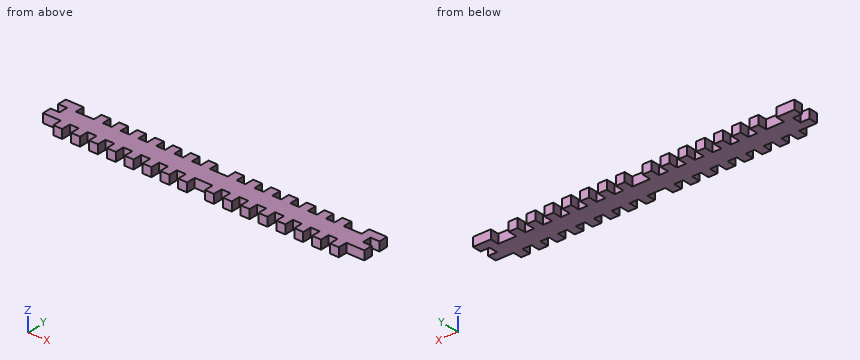
from build123d import *

# Parameters (mm, degrees)
BOSS_EXTRUDE1_DEPTH = 6.35


with BuildPart() as part:
    # Sketch1 → Boss-Extrude1 (new body)
    with BuildSketch(Plane.XY):
        Polygon((-107.95, 0), (-114.3, 0), (-114.3, -6.35), (-101.6, -6.35), (-101.6, -12.7), (-95.25, -12.7), (-95.25, -6.35), (-88.9, -6.35), (-88.9, -12.7), (-82.55, -12.7), (-82.55, -6.35), (-76.2, -6.35), (-76.2, -12.7), (-69.85, -12.7), (-69.85, -6.35), (-63.5, -6.35), (-63.5, -12.7), (-57.15, -12.7), (-57.15, -6.35), (-50.8, -6.35), (-50.8, -12.7), (-44.45, -12.7), (-44.45, -6.35), (-38.1, -6.35), (-38.1, -12.7), (-31.75, -12.7), (-31.75, -6.35), (-25.4, -6.35), (-25.4, -12.7), (-19.05, -12.7), (-19.05, -6.35), (-12.7, -6.35), (-12.7, -12.7), (-6.35, -12.7), (-6.35, -6.35), (0, -6.35), (6.35, -6.35), (6.35, -12.7), (12.7, -12.7), (12.7, -6.35), (19.05, -6.35), (19.05, -12.7), (25.4, -12.7), (25.4, -6.35), (31.75, -6.35), (31.75, -12.7), (38.1, -12.7), (38.1, -6.35), (44.45, -6.35), (44.45, -12.7), (50.8, -12.7), (50.8, -6.35), (57.15, -6.35), (57.15, -12.7), (63.5, -12.7), (63.5, -6.35), (69.85, -6.35), (69.85, -12.7), (76.2, -12.7), (76.2, -6.35), (82.55, -6.35), (82.55, -12.7), (88.9, -12.7), (88.9, -6.35), (95.25, -6.35), (95.25, -12.7), (101.6, -12.7), (101.6, -6.35), (114.3, -6.35), (114.3, 0), (107.95, 0), (107.95, 6.35), (114.3, 6.35), (114.3, 12.7), (107.95, 12.7), (101.6, 12.7), (101.6, 6.35), (95.25, 6.35), (88.9, 6.35), (88.9, 12.7), (82.55, 12.7), (82.55, 6.35), (76.2, 6.35), (76.2, 12.7), (69.85, 12.7), (69.85, 6.35), (63.5, 6.35), (63.5, 12.7), (57.15, 12.7), (57.15, 6.35), (50.8, 6.35), (50.8, 12.7), (44.45, 12.7), (44.45, 6.35), (38.1, 6.35), (38.1, 12.7), (31.75, 12.7), (31.75, 6.35), (25.4, 6.35), (25.4, 12.7), (19.05, 12.7), (19.05, 6.35), (12.7, 6.35), (12.7, 12.7), (6.35, 12.7), (6.35, 6.35), (0, 6.35), (-6.35, 6.35), (-6.35, 12.7), (-12.7, 12.7), (-12.7, 6.35), (-19.05, 6.35), (-19.05, 12.7), (-25.4, 12.7), (-25.4, 6.35), (-31.75, 6.35), (-31.75, 12.7), (-38.1, 12.7), (-38.1, 6.35), (-44.45, 6.35), (-44.45, 12.7), (-50.8, 12.7), (-50.8, 6.35), (-57.15, 6.35), (-57.15, 12.7), (-63.5, 12.7), (-63.5, 6.35), (-69.85, 6.35), (-69.85, 12.7), (-76.2, 12.7), (-76.2, 6.35), (-82.55, 6.35), (-82.55, 12.7), (-88.9, 12.7), (-88.9, 6.35), (-95.25, 6.35), (-101.6, 6.35), (-101.6, 12.7), (-107.95, 12.7), (-114.3, 12.7), (-114.3, 6.35), (-107.95, 6.35), align=None)
    extrude(amount=BOSS_EXTRUDE1_DEPTH)


solid = part.part
Design review of the part built by this model. Coordinates are the model's own, in mm. Coordinates: 2 decimals unless noted, no trailing zeros. Loops run counter-clockwise (first coordinate to the right, second up) from the corner with the lowest first, then second, coordinate; pieces in that order, holes last. Notation, with made-up numbers: (32.5, 72) - (42.5, 72) arc R14 ccw to (42.5, 93) - close; hole circle Ø9 at (82.25, -13.5). An arc over 180 degrees is marked (long way). Use CSV: the item, a comma, the result in double quotes. Start each with the question number.
1. To check wall thickness, follow probe 1 along X at (y, z) = (2, 2); probe 2 along Y at (x, z) = (-99.5, 2.5); probe 3 along Y at (x, z) = (-15, 4.75). State the ranges of each line that lie inside material, in increasing order.
2. Clearance check with flat-ended pins moving along their axes: pin 1 (1.9 mm diameter, centred on x = 91, z = 2, fed in from -Y); pin 2 (3 mm diameter, centred on y = -9, z = 3.5, fed in from -X); pin 3 (1 mm diameter, centred on y = 5.5, z = 3, fed in from +X). State where each tip first meets the part, or that it passes through.
3. Add section A-A on y = 8.75. Count the separate pieces of the cut face and the enclosed holes in it, plus the area to 3 significant figures.
4. Add section B-B on x = 53.5. Give the boundary of the cut face in (y, z).
Resolved:
1,probe 1,"-107.95 to 107.95"
1,probe 2,"-12.7 to 6.35"
1,probe 3,"-6.35 to 6.35"
2,pin 1,"y = -6.35"
2,pin 2,"x = -101.6"
2,pin 3,"x = 107.95"
3,separate pieces,"16"
3,enclosed holes,"0"
3,area,"726 mm2"
4,outline,"(-6.35, 0) - (6.35, 0) - (6.35, 6.35) - (-6.35, 6.35) - close"
